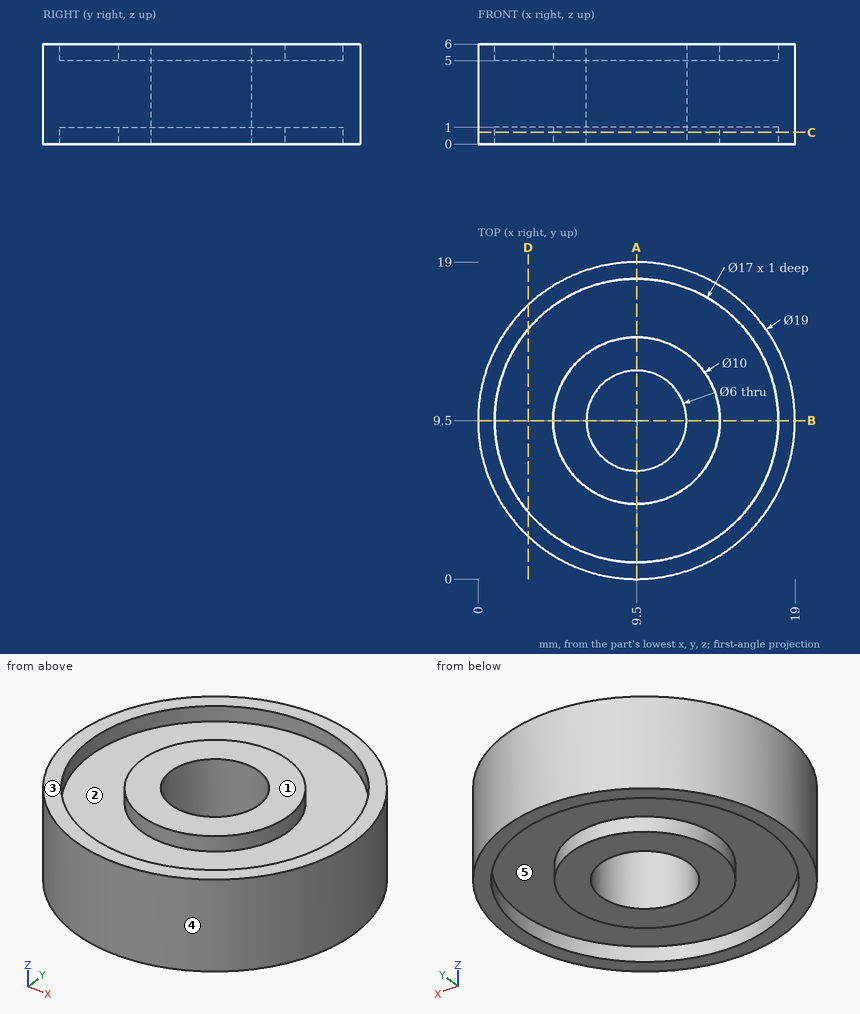
Study the drawing (mm; zero at the part's minimum x, y, z) and answer. A direction names the side the tool comes from. Round coordinates to 2 decimals unless told otherwise and drop trailing zeros. Loops run counter-clockwise (first coordinate to the right, second up) from the corner with the lowest first, then second, coordinate; pieces in that order, holes last. Notation, with made-up numbers: M 81.25,-35 L 126.25,-35 A24 ccw 126.25,-18 Z; hole C -0.5,-4.75 d11. An arc over 180 degrees is marked long. One line per question, with ' | ' between items.
Q1. A tool of negligible diameter and unlimited length cuts with its end or side. For the marked faces 1 and 2, from which of +Z, -Z, +X, -X, +Y, -Y can it reach the whole face along a straight path? Write none if from no direction.
Conclusion:
face 1: +Z, +X, -X, +Y, -Y | face 2: +Z
Q2. Find section C-C, the plane z = 0.7. Give the vertices of the cut face in (x, y).
Conclusion:
outline: C 9.5,9.5 d19; C 9.5,9.5 d10; hole C 9.5,9.5 d17; hole C 9.5,9.5 d6
Q3. Consider line 1 along Y through (x, z) = (9.5, 0.5); line 2 along Y through (x, z) = (8.5, 0.6); line 3 along Z through (x, y) = (16, 11.5). Determine where each line is inside the solid, lowest interval first. Write a range as from..to.
Conclusion:
line 1: y = 0..1, 4.5..6.5, 12.5..14.5, 18..19 | line 2: y = 0.05..1.06, 4.6..6.67, 12.33..14.4, 17.94..18.95 | line 3: z = 1..5
Q4. Find section D-D, the plane x = 3. Give the vertices of the cut face in (y, z), then the cut area to 3 significant figures.
Conclusion:
outline: M 2.57,0 L 4.02,0 L 4.02,1 L 14.98,1 L 14.98,0 L 16.43,0 L 16.43,6 L 14.98,6 L 14.98,5 L 4.02,5 L 4.02,6 L 2.57,6 Z | area: 61.2 mm2
Q5. Each of these flat-tipped pins is pushed along its axis until it touches: pin 1 Ø1 at (y, z) = (10.5, 2.5) entering from +X; pin 2 Ø2 at (y, z) = (13, 5) entering from +X. Where does it stop, or does it pass through?
Conclusion:
pin 1: stops at x = 18.99 | pin 2: stops at x = 18.67
Q6. Find section A-A, the plane x = 9.5. Give the vertices of the cut face in (y, z).
Conclusion:
outline: M 0,0 L 1,0 L 1,1 L 4.5,1 L 4.5,0 L 6.5,0 L 6.5,6 L 4.5,6 L 4.5,5 L 1,5 L 1,6 L 0,6 Z; M 12.5,0 L 14.5,0 L 14.5,1 L 18,1 L 18,0 L 19,0 L 19,6 L 18,6 L 18,5 L 14.5,5 L 14.5,6 L 12.5,6 Z
Q7. The mould has two halves that part along X. Classify the marked faces 3, 4 and 5: +X half, -X half, draft (parallel to the pull), parting line (faces both ways), or undercut.
Conclusion:
face 3: draft | face 4: parting line | face 5: undercut
